Model file for the job. Use its own axes, mm. Round coordinates to 2 decimals unless told otherwise and drop trailing zeros. Write each loop counter-clockwise with the first axis right and the second up, starting at its lowest first coordinate (ties: lowest second). Pieces come first, ordered by that corner, then holes.
```python
from build123d import *

# Parameters (mm, degrees)
SKETCH1_W           = 50
SKETCH1_H           = 120
BOSS_EXTRUDE1_DEPTH = 2
SKETCH2_W           = 0.5
SKETCH2_H           = 5.295420769
SKETCH2_H_2         = 23.549654675
BOSS_EXTRUDE3_DEPTH = 1


with BuildPart() as part:
    # Sketch1 → Boss-Extrude1 (new body)
    with BuildSketch(Plane(origin=(0, 0, 0), x_dir=(1, 0, 0), z_dir=(0, 1, 0))):
        with Locations((25, 60)):
            Rectangle(SKETCH1_W, SKETCH1_H)
    extrude(amount=BOSS_EXTRUDE1_DEPTH)

    # Sketch2 → Boss-Extrude3 (add)
    with BuildSketch(Plane(origin=(0, 2, 0), x_dir=(1, 0, 0), z_dir=(0, 1, 0))):
        with BuildLine():
            Line((9.849958258, 39.051579924), (16.845127039, 39.051579924))
            Line((16.845127039, 39.051579924), (16.845127039, 40.051579924))
            Line((16.845127039, 40.051579924), (10.349958258, 40.051579924))
            Line((10.349958258, 40.051579924), (10.349958258, 39.551579924))
            ThreePointArc((10.349958258, 39.551579924), (10.203511648, 39.198026534), (9.849958258, 39.051579924))
        make_face()
        with BuildLine():
            Line((10.349958258, 40.051579924), (10.349958258, 86.455511816))
            Line((10.349958258, 86.455511816), (9.849958258, 86.455511816))
            ThreePointArc((9.849958258, 86.455511816), (9.496404867, 86.601958426), (9.349958258, 86.955511816))
            Line((9.349958258, 86.955511816), (9.349958258, 39.551579924))
            ThreePointArc((9.349958258, 39.551579924), (9.496404867, 39.198026534), (9.849958258, 39.051579924))
            ThreePointArc((9.849958258, 39.051579924), (10.203511648, 39.198026534), (10.349958258, 39.551579924))
            Line((10.349958258, 39.551579924), (10.349958258, 40.051579924))
        make_face()
        with BuildLine():
            Line((6.849958258, 33.630782095), (16.845127039, 33.630782095))
            Line((16.845127039, 33.630782095), (16.845127039, 34.630782095))
            Line((16.845127039, 34.630782095), (7.349958258, 34.630782095))
            Line((7.349958258, 34.630782095), (7.349958258, 92.250932585))
            Line((7.349958258, 92.250932585), (8.019263959, 92.250932585))
            ThreePointArc((8.019263959, 92.250932585), (8.37281735, 92.397379194), (8.519263959, 92.750932585))
            ThreePointArc((8.519263959, 92.750932585), (8.37281735, 93.104485976), (8.019263959, 93.250932585))
            Line((8.019263959, 93.250932585), (7.349958258, 93.250932585))
            Line((7.349958258, 93.250932585), (7.349958258, 111.215314398))
            ThreePointArc((7.349958258, 111.215314398), (7.203511648, 111.568867789), (6.849958258, 111.715314398))
            ThreePointArc((6.849958258, 111.715314398), (6.496404867, 111.568867789), (6.349958258, 111.215314398))
            Line((6.349958258, 111.215314398), (6.349958258, 34.130782095))
            ThreePointArc((6.349958258, 34.130782095), (6.496404867, 33.777228705), (6.849958258, 33.630782095))
        make_face()
        with BuildLine():
            Line((9.849958258, 92.750932585), (10.349958258, 92.750932585))
            Line((10.349958258, 92.750932585), (10.349958258, 111.215314398))
            ThreePointArc((10.349958258, 111.215314398), (10.203511648, 111.568867789), (9.849958258, 111.715314398))
            ThreePointArc((9.849958258, 111.715314398), (9.496404867, 111.568867789), (9.349958258, 111.215314398))
            Line((9.349958258, 111.215314398), (9.349958258, 92.750932585))
            Line((9.349958258, 92.750932585), (9.849958258, 92.750932585))
        make_face()
        with Locations((10.099958258, 90.1032222)):
            Rectangle(SKETCH2_W, SKETCH2_H)
        with BuildLine():
            ThreePointArc((9.349958258, 86.955511816), (9.496404867, 87.309065207), (9.849958258, 87.455511816))
            Line((9.849958258, 87.455511816), (9.849958258, 92.750932585))
            Line((9.849958258, 92.750932585), (9.349958258, 92.750932585))
            Line((9.349958258, 92.750932585), (9.349958258, 86.955511816))
        make_face()
        with BuildLine():
            ThreePointArc((11.055620389, 93.250932585), (10.702066998, 93.104485976), (10.555620389, 92.750932585))
            Line((10.555620389, 92.750932585), (23.349958258, 92.750932585))
            Line((23.349958258, 92.750932585), (23.349958258, 93.250932585))
            Line((23.349958258, 93.250932585), (11.055620389, 93.250932585))
        make_face()
        with BuildLine():
            Line((23.349958258, 92.750932585), (10.555620389, 92.750932585))
            ThreePointArc((10.555620389, 92.750932585), (10.702066998, 92.397379194), (11.055620389, 92.250932585))
            Line((11.055620389, 92.250932585), (23.849958258, 92.250932585))
            ThreePointArc((23.849958258, 92.250932585), (23.496404867, 92.397379194), (23.349958258, 92.750932585))
        make_face()
        with BuildLine():
            Line((10.349958258, 86.455511816), (25, 86.455511816))
            Line((25, 86.455511816), (26.849958258, 86.455511816))
            ThreePointArc((26.849958258, 86.455511816), (26.496404867, 86.601958426), (26.349958258, 86.955511816))
            Line((26.349958258, 86.955511816), (26.349958258, 87.455511816))
            Line((26.349958258, 87.455511816), (25, 87.455511816))
            Line((25, 87.455511816), (10.349958258, 87.455511816))
            Line((10.349958258, 87.455511816), (10.349958258, 86.455511816))
        make_face()
        with BuildLine():
            ThreePointArc((26.349958258, 86.955511816), (26.496404867, 86.601958426), (26.849958258, 86.455511816))
            ThreePointArc((26.849958258, 86.455511816), (27.203511648, 86.601958426), (27.349958258, 86.955511816))
            ThreePointArc((27.349958258, 86.955511816), (27.203511648, 87.309065207), (26.849958258, 87.455511816))
            Line((26.849958258, 87.455511816), (26.349958258, 87.455511816))
            Line((26.349958258, 87.455511816), (26.349958258, 86.955511816))
        make_face()
        with BuildLine():
            ThreePointArc((26.849958258, 87.455511816), (27.203511648, 87.309065207), (27.349958258, 86.955511816))
            Line((27.349958258, 86.955511816), (27.349958258, 111.005166491))
            ThreePointArc((27.349958258, 111.005166491), (26.849958258, 111.505166491), (26.349958258, 111.005166491))
            Line((26.349958258, 111.005166491), (26.849958258, 111.005166491))
            Line((26.849958258, 111.005166491), (26.849958258, 87.455511816))
        make_face()
        with Locations((26.599958258, 99.230339154)):
            Rectangle(SKETCH2_W, SKETCH2_H_2)
        with BuildLine():
            Line((23.849958258, 111.005166491), (23.849958258, 93.250932585))
            ThreePointArc((23.849958258, 93.250932585), (24.203511648, 93.104485976), (24.349958258, 92.750932585))
            Line((24.349958258, 92.750932585), (24.349958258, 111.005166491))
            Line((24.349958258, 111.005166491), (23.849958258, 111.005166491))
        make_face()
        with BuildLine():
            Line((23.349958258, 93.250932585), (23.349958258, 92.750932585))
            ThreePointArc((23.349958258, 92.750932585), (23.496404867, 92.397379194), (23.849958258, 92.250932585))
            ThreePointArc((23.849958258, 92.250932585), (24.203511648, 92.397379194), (24.349958258, 92.750932585))
            ThreePointArc((24.349958258, 92.750932585), (24.203511648, 93.104485976), (23.849958258, 93.250932585))
            Line((23.849958258, 93.250932585), (23.349958258, 93.250932585))
        make_face()
        with BuildLine():
            Line((23.349958258, 111.005166491), (23.349958258, 93.250932585))
            Line((23.349958258, 93.250932585), (23.849958258, 93.250932585))
            Line((23.849958258, 93.250932585), (23.849958258, 111.005166491))
            Line((23.849958258, 111.005166491), (24.349958258, 111.005166491))
            ThreePointArc((24.349958258, 111.005166491), (23.849958258, 111.505166491), (23.349958258, 111.005166491))
        make_face()
        with BuildLine():
            Line((9.849958258, 86.455511816), (10.349958258, 86.455511816))
            Line((10.349958258, 86.455511816), (10.349958258, 87.455511816))
            Line((10.349958258, 87.455511816), (9.849958258, 87.455511816))
            ThreePointArc((9.849958258, 87.455511816), (9.496404867, 87.309065207), (9.349958258, 86.955511816))
            ThreePointArc((9.349958258, 86.955511816), (9.496404867, 86.601958426), (9.849958258, 86.455511816))
        make_face()
    extrude(amount=BOSS_EXTRUDE3_DEPTH)


solid = part.part
```
1) Cut at D-D on x = 32.5. List the corners of the cut face in (y, z), and give its area (3 significant figures).
2) Flat gauge pins, fed straight in: pin 1 Ø0.8 at (y, z) = (2.5, -104) entering from +X; pin 2 Ø1.1 at (x, y) = (12.5, 2.5) entering from +Z; pin 3 Ø8 at (x, z) = (24.5, -82) entering from +Y; pin 4 Ø0.8 at (x, y) = (13.5, 2.5) entering from -Z. Where does each tip first touch, or does it go through?
3) Cut at B-B on x = 15.5. List the corners of the cut face in (y, z).
4) Wall check: probe 1 along Z at (x, y) = (13.5, 2.4); probe 2 along X at (y, z) = (2.3, -61); probe 3 along Y at (x, z) = (32, -78.5). Give the ranges that are in metal, low to high.
5) Cut at A-A on z = -77. List the corners of the cut face in (x, y).
6) Cut at C-C on z = -102. List the corners of the cut face in (x, y), and give its area (3 significant figures).
Result sheet:
1. outline: (0, -120) - (2, -120) - (2, 0) - (0, 0) - close
1. area: 240 mm2
2. pin 1: stops at x = 27.35
2. pin 2: stops at z = 0
2. pin 3: stops at y = 2
2. pin 4: stops at z = -93.25
3. outline: (0, -120) - (2, -120) - (2, -93.25) - (3, -93.25) - (3, -92.25) - (2, -92.25) - (2, -87.46) - (3, -87.46) - (3, -86.46) - (2, -86.46) - (2, -40.05) - (3, -40.05) - (3, -39.05) - (2, -39.05) - (2, -34.63) - (3, -34.63) - (3, -33.63) - (2, -33.63) - (2, 0) - (0, 0) - close
4. probe 1: z = -93.25 to -92.25, -87.46 to -86.46, -40.05 to -39.05, -34.63 to -33.63
4. probe 2: x = 6.35 to 7.35, 9.35 to 10.35
4. probe 3: y = 0 to 2
5. outline: (0, 0) - (50, 0) - (50, 2) - (10.35, 2) - (10.35, 3) - (9.35, 3) - (9.35, 2) - (7.35, 2) - (7.35, 3) - (6.35, 3) - (6.35, 2) - (0, 2) - close
6. outline: (0, 0) - (50, 0) - (50, 2) - (27.35, 2) - (27.35, 3) - (26.35, 3) - (26.35, 2) - (24.35, 2) - (24.35, 3) - (23.35, 3) - (23.35, 2) - (10.35, 2) - (10.35, 3) - (9.35, 3) - (9.35, 2) - (7.35, 2) - (7.35, 3) - (6.35, 3) - (6.35, 2) - (0, 2) - close
6. area: 104 mm2
